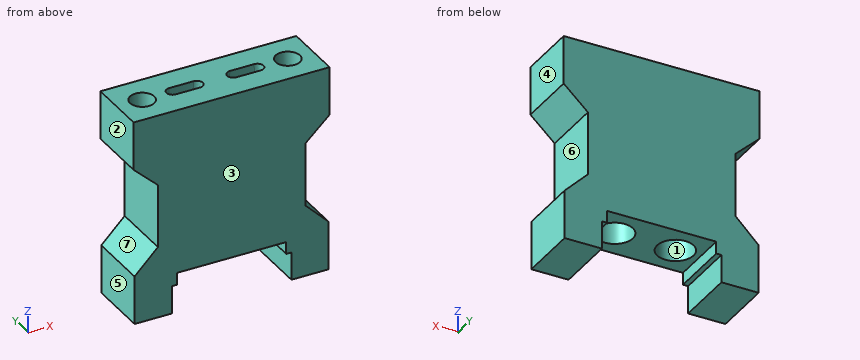
from build123d import *

# Parameters (mm, degrees)
SKETCH060_R     = 2.7
PAD029_DEPTH    = 10
SKETCH057_R     = 2.6
POCKET022_DEPTH = 18
SKETCH058_R     = 3
POCKET023_DEPTH = 10
SKETCH061_R     = 2
POCKET024_DEPTH = 8


with BuildPart() as loft002:
    # Sketch060 → Loft002 section 0
    with BuildSketch(Plane.XY.offset(28)):
        with Locations((-5, 0)):
            Circle(SKETCH060_R)
    # Sketch059 → Loft002 section 1
    with BuildSketch(Plane.XY.offset(38)):
        with BuildLine():
            ThreePointArc((-7, 1), (-8, 0), (-7, -1))
            Line((-7, -1), (-3, -1))
            ThreePointArc((-3, -1), (-2, 0), (-3, 1))
            Line((-3, 1), (-7, 1))
        make_face()
    loft()


with BuildPart() as part_mirroring002:
    # Part__Mirroring002: instance of Loft002
    add(loft002.part.mirror(Plane(origin=(0, 0, 0), x_dir=(0, -1, 0), z_dir=(1, 0, 0))))


with BuildPart() as fusion002:
    # Fusion002 base: copy of Loft002
    add(loft002.part)

    # Fusion002: union Part__Mirroring002
    add(part_mirroring002.part)


with BuildPart() as sensor_holder_sun:
    # Sketch056 → Pad029 (new body)
    with BuildSketch(Plane.XZ):
        Polygon((-16, 4), (-9.85, 4), (-9.85, 7), (-9.85, 8.6), (-9, 8.6), (-9, 10.6), (9, 10.6), (9, 8.6), (9.85, 8.6), (9.85, 7), (9.85, 4), (16, 4), (16, 12), (12.15, 15.85), (12.15, 26.306086), (16.15, 30), (16.15, 38), (-16.15, 38), (-16.15, 30), (-12.15, 26.306086), (-12.15, 15.85), (-16, 12), align=None)
    extrude(amount=PAD029_DEPTH)

    # Sketch057 (on Face7 of Pad029) → Pocket022 (cut)
    with BuildSketch(Plane(origin=(0, 0, 10.6), x_dir=(1, 0, 0), z_dir=(0, 0, -1))):
        with Locations((-5, 5)):
            Circle(SKETCH057_R)
        with Locations((5, 5)):
            Circle(SKETCH057_R)
    extrude(amount=-POCKET022_DEPTH, mode=Mode.SUBTRACT)

    # Sketch058 (on Face11 of Pocket022) → Pocket023 (cut)
    with BuildSketch(Plane(origin=(0, 0, 10.6), x_dir=(1, 0, 0), z_dir=(0, 0, -1))):
        with Locations((-5, 5)):
            Circle(SKETCH058_R)
        with Locations((5, 5)):
            Circle(SKETCH058_R)
    extrude(amount=-POCKET023_DEPTH, mode=Mode.SUBTRACT)

    # Sketch061 (on Face22 of Pocket023) → Pocket024 (cut)
    with BuildSketch(Plane(origin=(0, 0, 38), x_dir=(-1, 0, 0), z_dir=(0, 0, 1))):
        with Locations((-12, 5)):
            Circle(SKETCH061_R)
        with Locations((12, 5)):
            Circle(SKETCH061_R)
    extrude(amount=-POCKET024_DEPTH, mode=Mode.SUBTRACT)


with BuildPart() as sensor_holder_sun_1:
    # Body023 placement: moved
    add(sensor_holder_sun.part.moved(Location((0, 5, 0))))

    # Cut001: cut Fusion002
    add(fusion002.part, mode=Mode.SUBTRACT)


with BuildPart() as sensor_holder_sun_2:
    # Cut001 placement: moved
    add(sensor_holder_sun_1.part.moved(Location((0, -208.33, 0))))


solid = sensor_holder_sun_2.part
Design review of the part built by this model. Coordinates are the model's own, in mm. Face numbers are marked on the shaded views. A direction names the side the tool comes from. Coordinates: 2 decimals unless noted, no trailing zeros. Order: outer loops, then holes, each group sorted by start corner. A loop starts at its lowest first (then second) coordinate and runs counter-clockwise, first axis right, second up. Notation, with made-up numbers: (79.25, -34) -> (122.25, -34) arc R27 cw to (122.25, -9) -> close; hole circle Ø9 at (24.5, -22.75). An arc over 180 degrees is marked (long way). Use one line per item in the form item = value. Start each with the question number.
(1) The part is to be moulded in two halves that separate along X. For the marked faces 1, 2, 3 and 4, say which applies: +X half, -X half, draft (parallel to the pull), parting line (faces both ways), or undercut.
(2) For probe 1 along X at (y, z) = (-208.33, 16.5); probe 2 along X at (y, z) = (-208.33, 26); probe 3 along Y at (x, z) = (5, 18.5), list the stretches that pass through material, from the lowest coordinate up.
(3) Add section A-A on x = -10.5. State the section outline as (y, z) points.
(4) Add section C-C on x = 11. State the section outline as (y, z) points, plus the area to 3 significant figures.
(5) For the marked faces 5, 6 and 7, list the 3-axis set-ups (+Z, -Z, +X, -X, +Y, -Y) from which the entire face can be reached by the end or side of a thin tool; tool diameter is ignored.
(6) Add section B-B on z = 32.5. Give the number of separate pieces and of enclosed holes in the cut face, plus the area to 3 significant figures.
(7) Add section D-D on x = 0.5. State the section outline as (y, z) points.
(8) Insertion check: pin 1 (6 mm diameter, centred on y = -209, z = 7.5, fed in from -X); pin 2 (3 mm diameter, centred on x = -5, y = -207, fed in from -Z); pin 3 (0.6 mm diameter, centred on y = -210.5, z = 10, fed in from +X). Each pin has a flat end and moves straight along its axis. Give the tip position at first contact, or say it passes through.
Answer block:
q1.face_1 = undercut
q1.face_2 = -X half
q1.face_3 = draft
q1.face_4 = +X half
q2.probe_1 = -12.15 to -8, -2 to 2, 8 to 12.15
q2.probe_2 = -12.15 to -7.6, -2.4 to 2.4, 7.6 to 12.15
q2.probe_3 = -213.33 to -211.33, -205.33 to -203.33
q3.outline = (-213.33, 4) -> (-203.33, 4) -> (-203.33, 38) -> (-207.01, 38) -> (-207.01, 30) -> (-209.65, 30) -> (-209.65, 38) -> (-213.33, 38) -> close
q4.outline = (-213.33, 4) -> (-203.33, 4) -> (-203.33, 38) -> (-206.6, 38) -> (-206.6, 30) -> (-210.06, 30) -> (-210.06, 38) -> (-213.33, 38) -> close
q4.area = 312 mm²
q5.face_5 = -Z, -X, +Y, -Y
q5.face_6 = +X, +Y, -Y
q5.face_7 = -X, +Y, -Y
q6.separate_pieces = 1
q6.enclosed_holes = 4
q6.area = 264 mm²
q7.outline = (-213.33, 10.6) -> (-203.33, 10.6) -> (-203.33, 38) -> (-213.33, 38) -> close
q8.pin_1 = -16
q8.pin_2 = 20.6
q8.pin_3 = 16
